Autodesk Inventor part; units mm, degrees
ref_plane "YZ Plane" through (0, 0, 0) normal (1, 0, 0) x (0, 1, 0)
ref_plane "XZ Plane" through (0, 0, 0) normal (0, 1, 0) x (-1, 0, 0)
ref_plane "XY Plane" through (0, 0, 0) normal (0, 0, 1) x (1, 0, 0)
sketch "Sketch1" plane through (0, 0, 0) normal (0, 0, 1) x (1, 0, 0)
  line L0 (15.2673, 33.0721) -> (15.2673, -66.9279) construction
  line L1 (7.7673, 33.0721) -> (7.7673, -66.9279)
  line L2 (22.7673, -66.9279) -> (22.7673, 33.0721)
  arc A0 (22.7673, 33.0721) -> (7.7673, 33.0721) centre (15.2673, 33.0721) ccw
  arc A1 (7.7673, -66.9279) -> (22.7673, -66.9279) centre (15.2673, -66.9279) ccw
  circle A2 centre (15.2673, 33.0721) radius 2.5
  circle A3 centre (15.2673, -66.9279) radius 2.5
  point P0 (0, 0)
  point P1 (15.2673, -16.9279)
  dimension "d0" = 100
  dimension "d1" = 15
  dimension "d2" = 5
extrude "Extrusion1" add sketch "Sketch1" along normal blind 4
sketch "Sketch2" plane through (0, 0, 4) normal (0, 0, 1) x (1, 0, 0)
  point P0 (0, 0)
properties part number "2nd_part[1]"
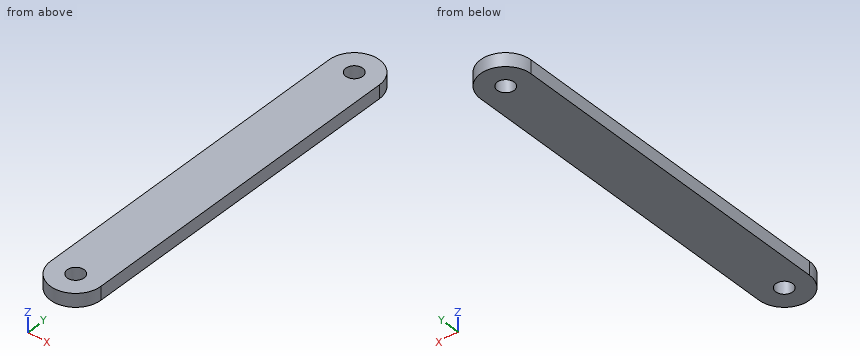
The model under review builds one solid part; all positions refer to its coordinate system, in mm. Round coordinates to 2 decimals unless told otherwise and drop trailing zeros. Loops run counter-clockwise (first coordinate to the right, second up) from the corner with the lowest first, then second, coordinate; pieces in that order, holes last.
1) Consider section C-C on x = 11. State the section outline as (y, z) points.
Values follow:
outline: (-73.1, 0) - (39.24, 0) - (39.24, 4) - (-73.1, 4) - close
2) Wall thickness on line 1 along Y through (x, z) = (17.5, 3.5); line 2 along Y through (x, z) = (15.25, 2.1); line 3 along X through (y, z) = (-69, 0.5): over which ranges is each line inside the solid? List them lowest first.
Values follow:
line 1: y = -74.09 to -68.05, -65.8 to 31.95, 34.2 to 40.23
line 2: y = -74.43 to -69.43, -64.43 to 30.57, 35.57 to 40.57
line 3: x = 8.06 to 13.87, 16.67 to 22.48
3) Clearance check with flat-ended pins moving along their axes: P1, Ø2, axis at x = 9.5, z = 3.5, coming from the -Y side; P2, Ø1, axis at x = 18, z = 1, coming from the -Y side. State where each tip first meets the part, or that it passes through.
Values follow:
P1: stops at y = -72.72
P2: stops at y = -74.09
4) Consider section B-B on x = 21.5. State the section outline as (y, z) points, then the cut area to 3 significant figures.
Values follow:
outline: (-71.1, 0) - (37.24, 0) - (37.24, 4) - (-71.1, 4) - close
area: 433 mm2
5) Consider section A-A on z = 2.65. State the section outline as (x, y) points, then the cut area to 3 significant figures.
Values follow:
outline: (7.77, -66.93) arc R7.5 ccw to (22.77, -66.93) - (22.77, 33.07) arc R7.5 ccw to (7.77, 33.07) - close; hole circle Ø5 at (15.27, -66.93); hole circle Ø5 at (15.27, 33.07)
area: 1,640 mm2
